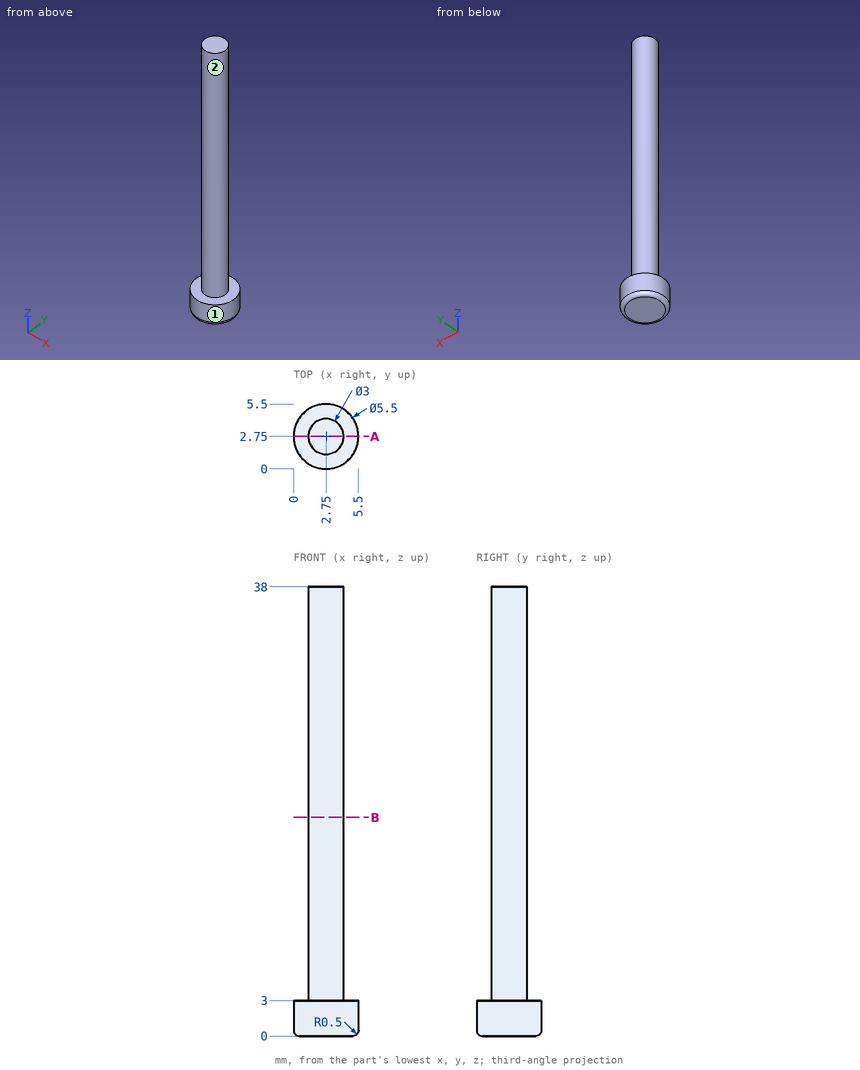
Geometry check sheet. Reference: drawing and pictorial views, mm from the part's lowest x, y, z. A direction names the side the tool comes from. Round coordinates to 2 decimals unless told otherwise and drop trailing zeros. Write each loop counter-clockwise with the first axis right and the second up, starting at its lowest first coordinate (ties: lowest second). Pieces come first, ordered by that corner, then holes.
(1) Material ranges on line 1 (Z direction, x = 2.45, y = 5.05); line 2 (Y direction, x = 2.65, z = 25); line 3 (Z direction, x = 4.2, y = 0.6), recorded low to high.
Returned:
line 1: z = 0 to 3
line 2: y = 1.25 to 4.25
line 3: z = 0.14 to 3
(2) Section check A-A (y = 2.75). Enter the section's corners in (x, z).
Returned:
outline: (0, 0.5) arc R0.5 ccw to (0.5, 0) - (5, 0) arc R0.5 ccw to (5.5, 0.5) - (5.5, 3) - (4.25, 3) - (4.25, 38) - (1.25, 38) - (1.25, 3) - (0, 3) - close
(3) Depth check by flat-ended pin: pin 1 Ø3 at (x, z) = (4.5, 5) entering from -Y; pin 2 Ø2 at (y, z) = (1.5, 29) entering from +X; pin 3 Ø1 at (x, y) = (2, 2) entering from -Z. Enter the tip coordinate at first touch or a pass-through.
Returned:
pin 1: stops at y = 1.27
pin 2: stops at x = 4.23
pin 3: stops at z = 0
(4) Section check B-B (z = 18.5). Enter the section's corners in (x, y), plus the area to 3 significant figures.
Returned:
outline: circle Ø3 at (2.75, 2.75)
area: 7.07 mm2
(5) Access from +Z, -Z, +X, -X, +Y, -Y to the whole of each face (thin tool, end or side, straight path). Record for the marked faces 1 and 2.
Returned:
face 1: +Z, -Z
face 2: +Z
